Read the model definition and answer for the solid it produces. Units are mm, in the model's axes. Coordinates: 2 decimals unless noted, no trailing zeros. Order: outer loops, then holes, each group sorted by start corner. A loop starts at its lowest first (then second) coordinate and runs counter-clockwise, first axis right, second up. Notation, with made-up numbers: (-4.75, 26) -> (31.25, 26) arc R9 cw to (31.25, 38) -> close; hole circle Ø10 at (52.5, 27). An arc over 180 degrees is marked (long way). Answer in a Markdown table with one row per item.
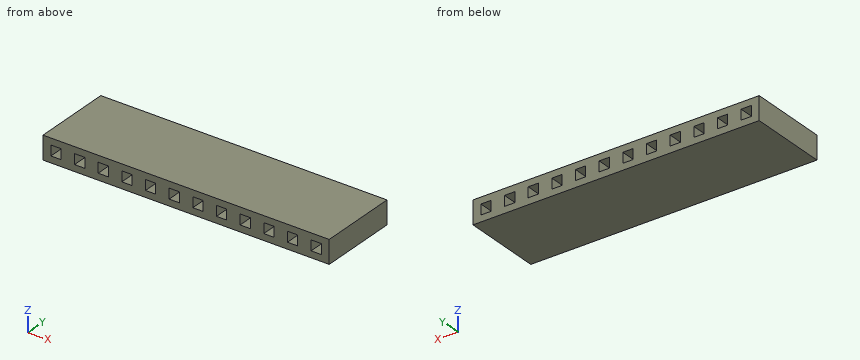
from build123d import *

# Parameters (mm, degrees)
SKETCH1_W           = 30.73
SKETCH1_H           = 8.5
BOSS_EXTRUDE1_DEPTH = 1.25
SKETCH2_W           = 1.1
SKETCH2_H           = 1.1
CUT_EXTRUDE1_DEPTH  = 32.908390746


with BuildPart() as part:
    # Sketch1 → Boss-Extrude1 (new, symmetric)
    with BuildSketch(Plane.XY):
        with Locations((15.365, 4.25)):
            Rectangle(SKETCH1_W, SKETCH1_H)
    extrude(amount=BOSS_EXTRUDE1_DEPTH, both=True)

    # Sketch2 → Cut-Extrude1 (cut, through all)
    with BuildSketch(Plane.XZ):
        with Locations((3.935, 0)):
            Rectangle(SKETCH2_W, SKETCH2_H)
        with Locations((1.395, 0)):
            Rectangle(SKETCH2_W, SKETCH2_H)
        with Locations((6.475, 0)):
            Rectangle(SKETCH2_W, SKETCH2_H)
        with Locations((9.015, 0)):
            Rectangle(SKETCH2_W, SKETCH2_H)
        with Locations((11.555, 0)):
            Rectangle(SKETCH2_W, SKETCH2_H)
        with Locations((14.095, 0)):
            Rectangle(SKETCH2_W, SKETCH2_H)
        with Locations((16.635, 0)):
            Rectangle(SKETCH2_W, SKETCH2_H)
        with Locations((19.175, 0)):
            Rectangle(SKETCH2_W, SKETCH2_H)
        with Locations((21.715, 0)):
            Rectangle(SKETCH2_W, SKETCH2_H)
        with Locations((24.255, 0)):
            Rectangle(SKETCH2_W, SKETCH2_H)
        with Locations((26.795, 0)):
            Rectangle(SKETCH2_W, SKETCH2_H)
        with Locations((29.335, 0)):
            Rectangle(SKETCH2_W, SKETCH2_H)
    extrude(amount=-CUT_EXTRUDE1_DEPTH, mode=Mode.SUBTRACT)


solid = part.part
Q1. The part is cut by section A-A (x = 6.5). Write down the section's boundary in (y, z), then the cut area to 3 significant figures.
Outcome:
| item | result |
|---|---|
| outline | (0, -1.25) -> (8.5, -1.25) -> (8.5, -0.55) -> (0, -0.55) -> close; (0, 0.55) -> (8.5, 0.55) -> (8.5, 1.25) -> (0, 1.25) -> close |
| area | 11.9 mm² |
Q2. The part is cut by section B-B (z = -0.1). Give the number of separate pieces and of enclosed holes in the cut face, then the cut area to 3 significant figures.
Outcome:
| item | result |
|---|---|
| separate pieces | 13 |
| enclosed holes | 0 |
| area | 149 mm² |
Q3. Consider line 1 (Z direction, x = 14, y = 1.5). Determine where the line is inside the solid, lowest interval first.
Outcome:
| item | result |
|---|---|
| line 1 | -1.25 to -0.55, 0.55 to 1.25 |
